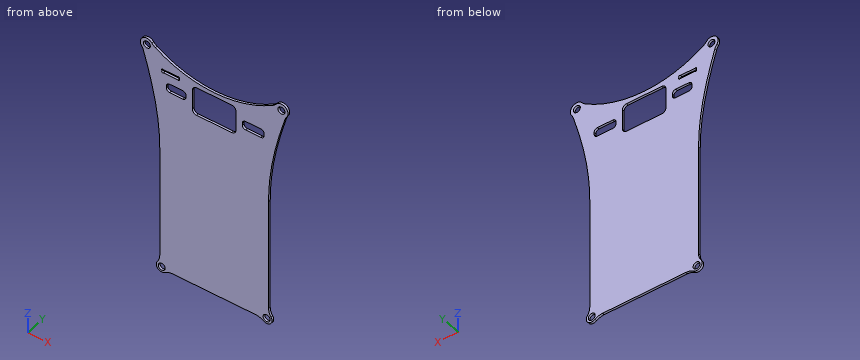
```python
from build123d import *

# Parameters (mm, degrees)
COVER_MAIN_BOARD_1_START = 30
COVER_MAIN_BOARD_1_DEPTH = 1
SKETCH_2_R               = 2.5
SKETCH_2_R_2             = 3
EXTRUDE_1_DEPTH          = 1
FILLET_1_R               = 6
HOLE_WIZARD_M31_D        = 3.2
SKETCH_5_W               = 20
SKETCH_5_H               = 13
CUT_EXTRUDE_2_DEPTH      = 118.861812366
FILLET_2_R               = 2
CUT_EXTRUDE_3_DEPTH      = 118.861812366
SKETCH_7_W               = 10
SKETCH_7_H               = 4
SKETCH_7_W_2             = 9
CUT_EXTRUDE_4_DEPTH      = 118.861812366
FILLET_3_R               = 1.5


# Read off the part's stored shape, not the designer's step: Припуск-Cover_main_board-1
with BuildPart() as part:
    # Припуск-Cover_main_board-1 outline → Припуск-Cover_main_board-1 (new body)
    with BuildSketch(Plane(origin=(0, 0, 0), x_dir=(1, 0, 0), z_dir=(0, 1, 0)).offset(COVER_MAIN_BOARD_1_START)):
        with BuildLine():
            ThreePointArc((58.536662962, -97.610509717), (61.872887908, -97.542255565), (62.936422695, -94.379353532))
            add(Edge.make_bspline(
                [(62.936422695, -94.379353532), (61.798177223, -90.776493028), (60.72075986, -87.155811957), (58.774674414, -79.85329338), (57.908149184, -76.177190929), (56.466060339, -68.758031881), (55.893308454, -65.032046108), (55.109773151, -57.544971093), (54.899999704, -53.783069267), (54.9, -50)],
                knots=[0, 0, 0, 0, 0.25, 0.25, 0.5, 0.5, 0.75, 0.75, 1, 1, 1, 1], degree=3))
            Line((54.9, -50), (54.9, 6.4))
            Line((54.9, 6.4), (5.1, 6.4))
            Line((5.1, 6.4), (5.1, -50))
            add(Edge.make_bspline(
                [(5.1, -50), (5.099991031, -53.776486453), (4.890826579, -57.541590974), (4.10432522, -65.051764617), (3.53002006, -68.780548712), (2.088476888, -76.191600122), (1.222062078, -79.86132679), (-0.718312327, -87.143485068), (-1.7924779, -90.75713228), (-2.928662588, -94.354417399)],
                knots=[0, 0, 0, 0, 0.25, 0.25, 0.5, 0.5, 0.75, 0.75, 1, 1, 1, 1], degree=3))
            ThreePointArc((-2.928662588, -94.354417399), (-1.883263044, -97.534459074), (1.463338472, -97.610508751))
            ThreePointArc((1.463338472, -97.610508751), (30.000000864, -88.89999981), (58.536662962, -97.610509717))
        make_face()
    extrude(amount=COVER_MAIN_BOARD_1_DEPTH)

    # Эскиз2 → Бобышка-Вытянуть1 (add)
    with BuildSketch(Plane(origin=(0, 31, 0), x_dir=(1, 0, 0), z_dir=(0, 1, 0))):
        with Locations((6, 5.5)):
            Circle(SKETCH_2_R)
        with Locations((54, 5.5)):
            Circle(SKETCH_2_R)
        with Locations((-0.811267397, -96.088490424)):
            Circle(SKETCH_2_R_2)
        with Locations((60.811267397, -96.088490424)):
            Circle(SKETCH_2_R_2)
    extrude(amount=-EXTRUDE_1_DEPTH)

    # Скругление1
    fillet_1_edges = [part.edges().sort_by_distance(p)[0] for p in [
        (-2.75519034, 30.5, 93.803503862),
        (1.934506666, 30.5, 97.297094907),
        (58.065493335, 30.5, 97.297094908),
        (62.755023846, 30.5, 93.803362229),
        (54.9, 30.5, -3.167619242),
        (51.667619242, 30.5, -6.4),
        (8.332380758, 30.5, -6.4),
        (5.1, 30.5, -3.167619242),
    ]]
    fillet(fillet_1_edges, radius=FILLET_1_R)

    # Отверстие с зазором M31 (through all)
    with Locations(Plane(origin=(0, 31, 0), x_dir=(1, 0, 0), z_dir=(0, 1, 0))):
        with Locations((-0.811267397, -96.088490424), (60.811267397, -96.088490424), (54, 5.5), (6, 5.5)):
            Hole(HOLE_WIZARD_M31_D / 2)

    # Эскиз5 → Вырез-Вытянуть2 (cut, through all)
    with BuildSketch(Plane.XZ.offset(-30)):
        with Locations((30, 80.64999981)):
            Rectangle(SKETCH_5_W, SKETCH_5_H)
    extrude(amount=-CUT_EXTRUDE_2_DEPTH, mode=Mode.SUBTRACT)

    # Скругление2
    fillet_2_edges = [part.edges().sort_by_distance(p)[0] for p in [
        (40, 30.5, 87.14999981),
        (40, 30.5, 74.14999981),
        (20, 30.5, 74.14999981),
        (20, 30.5, 87.14999981),
    ]]
    fillet(fillet_2_edges, radius=FILLET_2_R)

    # Эскиз6 → Вырез-Вытянуть3 (cut, through all)
    with BuildSketch(Plane.XZ.offset(-30)):
        with BuildLine():
            Line((6.807106781, 88.05), (13.392893219, 88.05))
            ThreePointArc((13.392893219, 88.05), (14.1, 88.05), (14.1, 87.342893219))
            Line((14.1, 87.342893219), (14.1, 87.257106781))
            ThreePointArc((14.1, 87.257106781), (14.1, 86.55), (13.392893219, 86.55))
            Line((13.392893219, 86.55), (6.807106781, 86.55))
            ThreePointArc((6.807106781, 86.55), (6.1, 86.55), (6.1, 87.257106781))
            Line((6.1, 87.257106781), (6.1, 87.342893219))
            ThreePointArc((6.1, 87.342893219), (6.1, 88.05), (6.807106781, 88.05))
        make_face()
    extrude(amount=-CUT_EXTRUDE_3_DEPTH, mode=Mode.SUBTRACT)

    # Эскиз7 → Вырез-Вытянуть4 (cut, through all)
    with BuildSketch(Plane.XZ.offset(-30)):
        with Locations((47.9, 80.6)):
            Rectangle(SKETCH_7_W, SKETCH_7_H)
        with Locations((12.6, 80.6)):
            Rectangle(SKETCH_7_W_2, SKETCH_7_H)
    extrude(amount=-CUT_EXTRUDE_4_DEPTH, mode=Mode.SUBTRACT)

    # Скругление3
    fillet_3_edges = [part.edges().sort_by_distance(p)[0] for p in [
        (42.9, 30.5, 78.6),
        (42.9, 30.5, 82.6),
        (52.9, 30.5, 82.6),
        (52.9, 30.5, 78.6),
        (17.1, 30.5, 82.6),
        (17.1, 30.5, 78.6),
        (8.1, 30.5, 78.6),
        (8.1, 30.5, 82.6),
    ]]
    fillet(fillet_3_edges, radius=FILLET_3_R)


solid = part.part
```
Geometry check sheet. Reference: the model listing, model coordinates, mm. Round coordinates to 2 decimals unless told otherwise and drop trailing zeros. Loops run counter-clockwise (first coordinate to the right, second up) from the corner with the lowest first, then second, coordinate; pieces in that order, holes last. Notation, with made-up numbers: (45, 38) - (101, 38) arc R25 cw to (101, 73) - close; hole circle Ø8 at (-24, 27). An arc over 180 degrees is marked (long way). Use a Markdown table: item, result.
Q1. Cross-section at A-A on x = 29.5. Record the cut outline in (y, z).
Solutions:
| item | result |
|---|---|
| outline | (30, -6.4) - (31, -6.4) - (31, 74.15) - (30, 74.15) - close; (30, 87.15) - (31, 87.15) - (31, 88.9) - (30, 88.9) - close |
Q2. Go/stop test with flat-tipped pins: P1, Ø0.5, axis at x = 47, y = 30.5, coming from the -Z side; P2, Ø0.5, axis at y = 30.5, z = 82, coming from the -X side; P3, Ø0.5, axis at x = 9.5, y = 30.5, coming from the -Z side. Record where each tip stops, or that it passes through.
Solutions:
| item | result |
|---|---|
| P1 | stops at z = -6.4 |
| P2 | stops at x = 0.58 |
| P3 | stops at z = -6.65 |
Q3. Cross-section at C-C on y = 30.5. State how many separate pieces and enclosed holes the cut face has, plus the area to 3 significant figures.
Solutions:
| item | result |
|---|---|
| separate pieces | 1 |
| enclosed holes | 8 |
| area | 4,810 mm2 |
Q4. Cross-section at B-B on x = 36.5. Record the cut outline in (y, z).
Solutions:
| item | result |
|---|---|
| outline | (30, -6.4) - (31, -6.4) - (31, 74.15) - (30, 74.15) - close; (30, 87.15) - (31, 87.15) - (31, 89.32) - (30, 89.32) - close |
Q5. Material ranges on line 1 (X direction, y = 30.25, z = -5.5); line 2 (Z direction, x = 10, y = 30.75); line 3 (X direction, y = 30.95, z = 7), recorded low to high.
Solutions:
| item | result |
|---|---|
| line 1 | x = 3.5 to 4.4, 7.6 to 52.4, 55.6 to 56.5 |
| line 2 | z = -6.48 to 78.6, 82.6 to 86.55, 88.05 to 92.98 |
| line 3 | x = 5.1 to 54.9 |
